Build history of the part. All positions in model axes, mm. Give positions to 0.01 mm unless a question says otherwise; leave off trailing zeros. Order: outer loops, then holes, each group sorted by start corner. A loop starts at its lowest first (then second) coordinate and runs counter-clockwise, first axis right, second up. Notation, with made-up numbers: M 43.5,57 L 99.5,57 A14 cw 99.5,61 Z; hole C 83.25,85.25 d9. An arc over 180 degrees is marked long. Answer as CSV lines item,"result".
Autodesk Inventor part; units mm, degrees
ref_plane "YZ Plane" through (0, 0, 0) normal (1, 0, 0) x (0, 1, 0)
ref_plane "XZ Plane" through (0, 0, 0) normal (0, 1, 0) x (-1, 0, 0)
ref_plane "XY Plane" through (0, 0, 0) normal (0, 0, 1) x (1, 0, 0)
sketch "Sketch1" plane through (0, 0, 0) normal (0, 0, 1) x (1, 0, 0)
  circle A0 centre (-2.4288, -33.7476) radius 3.75 construction
  line L0 (-6.7056, -28.9306) -> (5.9944, -28.9306)
  line L1 (5.9944, -28.9306) -> (5.9944, -53.0606)
  line L2 (5.9944, -53.0606) -> (-6.7056, -53.0606)
  line L3 (-6.7056, -53.0606) -> (-6.7056, -28.9306)
  line L4 (9.1694, -22.5806) -> (-9.8806, -22.5806)
  line L5 (-9.8806, -22.5806) -> (-9.8806, -117.8306)
  line L6 (9.1694, -71.8398) -> (9.1694, -22.5806)
  line L7 (58.0161, -27.4833) -> (9.1694, -71.8398)
  line L8 (-9.8806, -117.8306) -> (53.7075, -54.2425) construction
  line L9 (115.843, 7.893) -> (102.3726, 21.3634) construction
  line L10 (102.3726, 21.3634) -> (71.3049, -9.7044) construction
  line L11 (5.9944, -38.1) -> (9.1694, -38.1) construction
  line L12 (-6.7056, -38.1) -> (-9.8806, -38.1) construction
  line L13 (53.7075, -54.2425) -> (40.2371, -40.7721) construction
  line L14 (53.7075, -54.2425) -> (84.7753, -23.1747) construction
  line L15 (40.2371, -40.7721) -> (9.1694, -71.8398) construction
  line L16 (84.7753, -23.1747) -> (71.3049, -9.7044) construction
  line L17 (21.9135, -86.0365) -> (9.1694, -71.8398) construction
  arc A1 (107.3117, 16.4242) -> (110.9038, 12.8321) centre (109.1078, 14.6282) ccw construction
  line L18 (84.7753, -23.1747) -> (115.843, 7.893) construction
  line L19 (71.3049, -9.7044) -> (40.2371, -40.7721) construction
  line L20 (69.2414, -38.7086) -> (55.771, -25.2382) construction
  line L21 (21.9135, -86.0365) -> (66.9963, -36.4636)
  line L22 (-9.8806, -117.8306) -> (21.9135, -86.0365)
  line L23 (66.9963, -36.4636) -> (110.9038, 12.8321)
  line L24 (58.0161, -27.4833) -> (107.3117, 16.4242)
  arc A2 (110.9038, 12.8321) -> (107.3117, 16.4242) centre (109.1078, 14.6282) ccw
  line L25 (2.1844, -28.9306) -> (-2.8956, -28.9306)
  line L26 (-2.8956, -28.9306) -> (-2.8956, -27.1526)
  line L27 (-2.8956, -27.1526) -> (2.1844, -27.1526)
  line L28 (2.1844, -27.1526) -> (2.1844, -28.9306)
  line L29 (5.6388, -37.0253) -> (5.6388, -52.2891)
  line L30 (5.4388, -52.4891) -> (-6.1612, -52.4891)
  dimension "d4" = 5.9944
  dimension "d5" = 5.9944
  dimension "d6" = 12.7
  dimension "d7" = 24.13
  dimension "d8" = 19.05
  dimension "d9" = 95.25
  dimension "d10" = 6.35
  dimension "d12" = 19.05
  dimension "d13" = 177.8
  dimension "d14" = 45
  dimension "d15" = 5.08
  dimension "d16" = 3.175
  dimension "d17" = 3.175
  dimension "d20" = 1.778
  dimension "d21" = 5.08
  dimension "d22" = 3.81
  dimension "d23" = 0.7056
  dimension "d24" = 0.5715
extrude "Extrusion1" add sketch "Sketch1" along normal blind 3.175
sketch "Sketch2" plane through (0, 0, 3.175) normal (0, 0, 1) x (1, 0, 0)
  arc A0 (-0.8612, -26.1231) -> (0.1388, -26.1231) centre (-0.3612, -26.9891) ccw
  arc A1 (0.1388, -55.8551) -> (-0.8612, -55.8551) centre (-0.3612, -54.9891) ccw
  circle A2 centre (-0.3612, -54.9891) radius 1
  circle A3 centre (-0.3612, -26.9891) radius 1
  point P0 (0, 0)
extrude "Extrusion2" cut sketch "Sketch2" against normal up to next
properties part number "Toe"
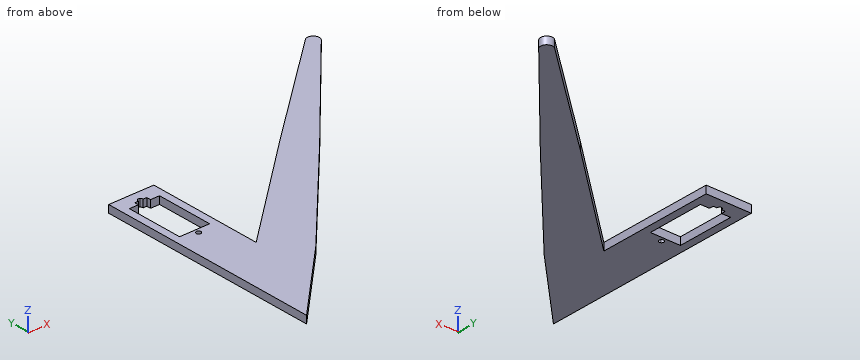
Item 1: Drop flat-ended pins along their axis: pin 1 (1 mm diameter, centred on y = -39, z = 2, fed in from +X); pin 2 (1.5 mm diameter, centred on x = 89, z = 2, fed in from +Y); pin 3 (0.9 mm diameter, centred on y = -28.5, z = 1, fed in from +X). Give the stop position or say it passes through.
Geometry says:
pin 1,"stops at x = 65.14"
pin 2,"stops at y = 0.78"
pin 3,"stops at x = 74.49"
Item 2: Band-saw the part on D-D (y = -43.5). Give the cut face in (x, z) (3 decimals).
Geometry says:
outline,"M -9.881,0 L -6.706,0 L -6.706,3.175 L -9.881,3.175 Z; M 5.994,0 L 9.169,0 L 9.169,3.175 L 5.994,3.175 Z; M 40.378,0 L 60.597,0 L 60.597,3.175 L 40.378,3.175 Z"
Item 3: Band-saw the part on A-A (x = 4.5). Give the cut face in (y, z) (3 decimals).
Geometry says:
outline,"M -103.45,0 L -53.061,0 L -53.061,3.175 L -103.45,3.175 Z; M -28.931,0 L -22.581,0 L -22.581,3.175 L -28.931,3.175 Z"
Item 4: Band-saw the part on B-B (y = -58). Give the cut face in (x, z) (3 decimals), and give its area (3 significant figures).
Geometry says:
outline,"M -9.881,0 L 9.169,0 L 9.169,3.175 L -9.881,3.175 Z; M 24.41,0 L 47.411,0 L 47.411,3.175 L 24.41,3.175 Z"
area,"134 mm2"
Item 5: Probe line 1 along X through (y, z) = (-35.5, 1.5); line 2 along Y through (x, z) = (1, 1.05); line 3 along X through (y, z) = (-23, 2). List the from-to ranges inside material, lowest first. Write a range as from..to.
Geometry says:
line 1,"x = -9.88..-6.71, 5.99..9.17, 49.19..67.85"
line 2,"y = -106.95..-53.06, -27.15..-22.58"
line 3,"x = -9.88..9.17, 63.05..78.99"
Item 6: Band-saw the part on C-C (z = 2.15). Give the cut face in (x, y).
Geometry says:
outline,"M -9.88,-117.83 L 21.91,-86.04 L 67,-36.46 L 110.9,12.83 A2.54 ccw 107.31,16.42 L 58.02,-27.48 L 9.17,-71.84 L 9.17,-22.58 L -9.88,-22.58 Z; hole M -6.71,-53.06 L 5.99,-53.06 L 5.99,-28.93 L 2.18,-28.93 L 2.18,-27.15 L 0.63,-27.15 A1 ccw 0.14,-26.12 A1 ccw -0.86,-26.12 A1 ccw -1.35,-27.15 L -2.9,-27.15 L -2.9,-28.93 L -6.71,-28.93 Z; hole M -0.86,-55.86 A1 ccw 0.14,-55.86 A1 ccw long Z"
